Autodesk Fusion 360 part; units mm, degrees
sketch "Sketch1" plane through (0, 0, 0) normal (0, 1, 0) x (1, 0, 0)
  line L0 (0, 0) -> (445, 0)
  line L1 (445, 0) -> (445, -500)
  line L2 (445, -500) -> (0, -500)
  line L3 (0, -500) -> (0, 0)
  dimension "d1" = 445
  dimension "d2" = 500
extrude "Extrude1" add sketch "Sketch1" along normal blind 50
ref_plane "WorkPlane1" through (222.5, 0, 250) normal (0, -1, 0) x (-1, 0, 0)
sketch "Sketch2" plane through (222.5, 0, 250) normal (0, -1, 0) x (1, 0, 0)
  line L0 (222.5, 250) -> (119.5, 250)
  line L1 (119.5, 250) -> (119.5, 237)
  line L2 (119.5, 237) -> (222.5, 237)
  line L3 (222.5, 237) -> (222.5, 250)
  line L4 (222.5, 250) -> (209.5, 250)
  line L5 (209.5, 250) -> (209.5, 147)
  line L6 (209.5, 147) -> (222.5, 147)
  line L7 (222.5, 147) -> (222.5, 250)
  line L8 (119.5, 237) -> (209.5, 147)
  line L9 (209.5, 237) -> (119.5, 237)
  line L10 (-222.5, 250) -> (-119.5, 250)
  line L11 (-119.5, 250) -> (-119.5, 237)
  line L12 (-119.5, 237) -> (-222.5, 237)
  line L13 (-222.5, 237) -> (-222.5, 250)
  line L14 (-222.5, 250) -> (-209.5, 250)
  line L15 (-209.5, 250) -> (-209.5, 147)
  line L16 (-209.5, 147) -> (-222.5, 147)
  line L17 (-222.5, 147) -> (-222.5, 250)
  line L18 (-222.5, -250) -> (-119.5, -250)
  line L19 (-119.5, -250) -> (-119.5, -237)
  line L20 (-119.5, -237) -> (-222.5, -237)
  line L21 (-222.5, -237) -> (-222.5, -250)
  line L22 (-222.5, -250) -> (-209.5, -250)
  line L23 (-209.5, -250) -> (-209.5, -147)
  line L24 (-209.5, -147) -> (-222.5, -147)
  line L25 (-222.5, -147) -> (-222.5, -250)
  line L26 (222.5, -250) -> (209.5, -250)
  line L27 (209.5, -250) -> (209.5, -147)
  line L28 (209.5, -147) -> (222.5, -147)
  line L29 (222.5, -147) -> (222.5, -250)
  line L30 (222.5, -250) -> (119.5, -250)
  line L31 (119.5, -250) -> (119.5, -237)
  line L32 (119.5, -237) -> (222.5, -237)
  line L33 (222.5, -237) -> (222.5, -250)
  line L34 (119.5, -237) -> (209.5, -147)
  line L35 (209.5, 147) -> (119.5, 237)
  line L36 (-119.5, 237) -> (-209.5, 147)
  line L37 (-209.5, -147) -> (-119.5, -237)
  line L38 (-209.5, 147) -> (-209.5, -147)
  line L39 (-119.5, -237) -> (119.5, -237)
  line L40 (209.5, 147) -> (209.5, -147)
  line L41 (119.5, 237) -> (-119.5, 237)
  dimension "d6" = 103
  dimension "d7" = 13
  dimension "d8" = 13
  dimension "d9" = 103
  dimension "d10" = 103
  dimension "d11" = 13
  dimension "d12" = 13
  dimension "d13" = 103
  dimension "d14" = 103
  dimension "d15" = 13
  dimension "d16" = 13
  dimension "d17" = 103
  dimension "d18" = 13
  dimension "d19" = 103
  dimension "d20" = 103
  dimension "d21" = 13
extrude "Extrude2" cut sketch "Sketch2" against normal blind 50 contours L8 L34 L35 L36 L37 L38 L39 L40 L41
ref_plane "WorkPlane2" through (442, 25, 250) normal (1, 0, 0) x (0, 0, -1)
sketch "Sketch3" plane through (442, 25, 250) normal (1, 0, 0) x (0, 1, 0)
  line L0 (-25, -250) -> (25, -250)
  line L1 (25, -250) -> (25, -247)
  line L2 (25, -247) -> (-25, -247)
  line L3 (-25, -247) -> (-25, -250)
  line L4 (-25, 250) -> (25, 250)
  line L5 (25, 250) -> (25, 247)
  line L6 (25, 247) -> (-25, 247)
  line L7 (-25, 247) -> (-25, 250)
  line L8 (-25, 247) -> (-22, 247)
  line L9 (-22, 247) -> (-22, -247)
  line L10 (-22, -247) -> (-25, -247)
  line L11 (-25, -247) -> (-25, 247)
  line L12 (-22, 247) -> (-19.4, 247)
  line L13 (-19.4, 247) -> (-19.4, 220.835)
  line L14 (-19.4, 220.835) -> (-22, 220.835)
  line L15 (-22, 220.835) -> (-22, 247)
  line L16 (-19.4, 247) -> (-16, 247)
  line L17 (-16, 247) -> (-16, -247)
  line L18 (-16, -247) -> (-19.4, -247)
  line L19 (-19.4, -247) -> (-19.4, 247)
  line L20 (-16, 247) -> (-13.4, 247)
  line L21 (-13.4, 247) -> (-13.4, 220.8212)
  line L22 (-13.4, 220.8212) -> (-16, 220.8212)
  line L23 (-16, 220.8212) -> (-16, 247)
  line L24 (-13.4, 247) -> (-10.4, 247)
  line L25 (-10.4, 247) -> (-10.4, -247)
  line L26 (-10.4, -247) -> (-13.4, -247)
  line L27 (-13.4, -247) -> (-13.4, 247)
  line L28 (-10.4, 247) -> (-7.8, 247)
  line L29 (-7.8, 247) -> (-7.8, 220.1918)
  line L30 (-7.8, 220.1918) -> (-10.4, 220.1918)
  line L31 (-10.4, 220.1918) -> (-10.4, 247)
  line L32 (-7.8, 247) -> (25, 247)
  line L33 (25, 247) -> (25, -247)
  line L34 (25, -247) -> (-7.8, -247)
  line L35 (-7.8, -247) -> (-7.8, 247)
  dimension "d25" = 3
  dimension "d26" = 50
  dimension "d27" = 3
  dimension "d28" = 3
  dimension "d29" = 2.6
  dimension "d30" = 3.4
  dimension "d31" = 2.6
  dimension "d32" = 3
  dimension "d33" = 2.6
extrude "Extrude3" cut sketch "Sketch3" against normal blind 439 contours L2 L6 L8 L9 L10 L11 L15 | L2 L6 L29 L32 L33 L34 L35 | L2 L6 L13 L16 L17 L18 L19 L23 | L2 L6 L21 L24 L25 L26 L27 L31
ref_plane "WorkPlane3" through (222.5, 50, 250) normal (0, 1, 0) x (0, 0, 1)
sketch "Sketch4" plane through (222.5, 50, 250) normal (0, 1, 0) x (1, 0, 0)
  line L0 (222.5, -250) -> (182.5, -250)
  line L1 (182.5, -250) -> (182.5, -210)
  line L2 (182.5, -210) -> (222.5, -210)
  line L3 (222.5, -210) -> (222.5, -250)
  line L4 (-222.5, -250) -> (-182.5, -250)
  line L5 (-182.5, -250) -> (-182.5, -210)
  line L6 (-182.5, -210) -> (-222.5, -210)
  line L7 (-222.5, -210) -> (-222.5, -250)
  line L8 (-222.5, 250) -> (-182.5, 250)
  line L9 (-182.5, 250) -> (-182.5, 210)
  line L10 (-182.5, 210) -> (-222.5, 210)
  line L11 (-222.5, 210) -> (-222.5, 250)
  line L12 (222.5, 250) -> (182.5, 250)
  line L13 (182.5, 250) -> (182.5, 210)
  line L14 (182.5, 210) -> (222.5, 210)
  line L15 (222.5, 210) -> (222.5, 250)
  dimension "d37" = 40
  dimension "d38" = 40
  dimension "d39" = 40
  dimension "d40" = 40
  dimension "d41" = 40
  dimension "d42" = 40
  dimension "d43" = 40
  dimension "d44" = 40
extrude "Extrude4" cut sketch "Sketch4" against normal blind 20
ref_plane "WorkPlane4" through (425, 30, 20) normal (0, 1, 0) x (0, 0, 1)
sketch "Sketch5" plane through (425, 30, 20) normal (0, 1, 0) x (1, 0, 0)
  line L0 (20, 20) -> (-20, 20)
  line L1 (-20, 20) -> (-20, -20)
  line L2 (-20, -20) -> (20, -20)
  line L3 (20, -20) -> (20, 20)
  line L4 (-425, 20) -> (-385, 20)
  line L5 (-385, 20) -> (-385, -20)
  line L6 (-385, -20) -> (-425, -20)
  line L7 (-425, -20) -> (-425, 20)
  line L8 (-425, -480) -> (-385, -480)
  line L9 (-385, -480) -> (-385, -440)
  line L10 (-385, -440) -> (-425, -440)
  line L11 (-425, -440) -> (-425, -480)
  line L12 (20, -480) -> (-20, -480)
  line L13 (-20, -480) -> (-20, -440)
  line L14 (-20, -440) -> (20, -440)
  line L15 (20, -440) -> (20, -480)
  dimension "d48" = 40
  dimension "d49" = 40
  dimension "d50" = 40
  dimension "d51" = 40
  dimension "d52" = 40
  dimension "d53" = 40
  dimension "d54" = 40
  dimension "d55" = 40
extrude "Extrude5" add sketch "Sketch5" against normal blind 13
ref_plane "WorkPlane5" through (222.5, 3, 250) normal (0, -1, 0) x (0, 0, 1)
sketch "Sketch6" plane through (222.5, 3, 250) normal (0, -1, 0) x (1, 0, 0)
ref_plane "WorkPlane6" through (425, 30, 480) normal (0, 1, 0) x (0, 0, 1)
sketch "Sketch7" plane through (425, 30, 480) normal (0, 1, 0) x (1, 0, 0)
  line L0 (20, -20) -> (0, -20)
  line L1 (0, -20) -> (0, 0)
  line L2 (0, 0) -> (20, 0)
  line L3 (20, 0) -> (20, -20)
  circle A0 centre (0, 0) radius 7.5
  line L4 (-425, -20) -> (-405, -20)
  line L5 (-405, -20) -> (-405, 0)
  line L6 (-405, 0) -> (-425, 0)
  line L7 (-425, 0) -> (-425, -20)
  circle A1 centre (-405, 0) radius 7.5
  line L8 (-425, 480) -> (-405, 480)
  line L9 (-405, 480) -> (-405, 460)
  line L10 (-405, 460) -> (-425, 460)
  line L11 (-425, 460) -> (-425, 480)
  circle A2 centre (-405, 460) radius 7.5
  line L12 (20, 480) -> (0, 480)
  line L13 (0, 480) -> (0, 460)
  line L14 (0, 460) -> (20, 460)
  line L15 (20, 460) -> (20, 480)
  circle A3 centre (0, 460) radius 7.5
  dimension "d60" = 20
  dimension "d61" = 20
  dimension "d62" = 15
  dimension "d63" = 20
  dimension "d64" = 20
  dimension "d65" = 15
  dimension "d66" = 20
  dimension "d67" = 20
  dimension "d68" = 15
  dimension "d69" = 20
  dimension "d70" = 20
  dimension "d71" = 15
extrude "Extrude6" cut sketch "Sketch7" against normal blind 2.65 contours L1 L2 A0 | L1 L2 A0 | L5 L6 A1 | L5 L6 A1 | L9 L10 A2 | L9 L10 A2 | L13 L14 A3 | L13 L14 A3
CAD build for the part. Positions are in the model's coordinates, mm. A direction names the side the tool comes from. Round coordinates to 2 decimals unless told otherwise and drop trailing zeros.
Q1. Which spindle directions (+Z, -Z, +X, -X, +Y, -Y) get a long thin tool onto all of the face, cutting with end or side? Do faces 1 (the flat face through (20, 27.35, 480)), 2 (the flat face through (57, 16, 59)), 3 (the flat face through (12, 14.6, 288)). Say none if no direction does.
Q2. Drop flat-ended pins along their axis: pin 1 (9 mm diameter, centred on x = 20, z = 20, fed in from -Y); pin 2 (3.5 mm diameter, centred on y = 43, z = 1, fed in from +X); pin 3 (12 mm diameter, centred on x = 22, z = 477, fed in from +Y). Give the stop position or say it passes through.
Q3. Wall check: L1, parallel to Z at x = 20, y = 28.2; L2, parallel to X at y = 29, z = 20; L3, parallel to Y at x = 27.5, z = 463. Give the ranges that are in metal, low to high.
Q4. Two-plate mould, pull along Y, no slides. Class faces 4 (the flat face through (12, 9, 288)), 5 (the flat face through (445, 25, 247)), 6 (the flat face through (416, 30, 20)): pulls with the +Y half, pulls with the -Y half, needs draft (parallel to the pull), parting line crosses it, or undercut.
Results below:
1. face 1: +Y
1. face 2: +Y, -Y
1. face 3: none
2. pin 1: stops at y = 3
2. pin 2: stops at x = 405
2. pin 3: stops at y = 30
3. L1: z = 0 to 12.5, 27.5 to 40, 460 to 472.5, 487.5 to 500
3. L2: x = 0 to 12.5, 27.5 to 40, 405 to 417.5, 432.5 to 445
3. L3: y = 3 to 5.6, 9 to 11.6, 14.6 to 30
4. face 4: undercut
4. face 5: needs draft
4. face 6: pulls with the +Y half
